The model under review builds one solid part; all positions refer to its coordinate system, in mm. A direction names the side the tool comes from. Give positions to 0.01 mm unless a question says otherwise; leave off trailing zeros. Order: outer loops, then holes, each group sorted by start corner. A loop starts at its lowest first (then second) coordinate and runs counter-clockwise, first axis right, second up. Notation, with made-up numbers: (-4.5, -10) - (36.5, -10) arc R9 ccw to (36.5, -1) - close; hole circle Ø3 at (49, -0.5). An arc over 180 degrees is marked (long way). Use CSV: the item, a comma, the result in double quotes.
```python
from build123d import *

# Parameters (mm, degrees)
SKETCH_1_W          = 300
SKETCH_1_H          = 370
EXTRUDE_1_DEPTH     = 10
SKETCH_2_R          = 1.5
SKETCH_2_R_2        = 2
SKETCH_2_W          = 25
SKETCH_2_H          = 34
CUT_EXTRUDE_1_DEPTH = 10


with BuildPart() as part:
    # 草图1 → 凸台-拉伸1 (new body)
    with BuildSketch(Plane.XY):
        with Locations((113.99815703, 205.554685433)):
            Rectangle(SKETCH_1_W, SKETCH_1_H)
    extrude(amount=EXTRUDE_1_DEPTH)

    # 草图2 → 切除-拉伸1 (cut)
    with BuildSketch(Plane.XY.offset(10)):
        with Locations((253.99815703, 375.554685433)):
            Circle(SKETCH_2_R)
        with Locations((253.99815703, 337.554685433)):
            Circle(SKETCH_2_R)
        with Locations((-26.00184297, 337.554685433)):
            Circle(SKETCH_2_R)
        with Locations((-26.00184297, 375.554685433)):
            Circle(SKETCH_2_R)
        with Locations((-26.00184297, 35.554685433)):
            Circle(SKETCH_2_R)
        with Locations((-26.00184297, 73.554685433)):
            Circle(SKETCH_2_R)
        with Locations((253.99815703, 73.554685433)):
            Circle(SKETCH_2_R)
        with Locations((253.99815703, 35.554685433)):
            Circle(SKETCH_2_R)
        with Locations((237.99815703, 355.804685433)):
            Circle(SKETCH_2_R)
        with Locations((-10.00184297, 355.804685433)):
            Circle(SKETCH_2_R)
        with Locations((-10.00184297, 55.304685433)):
            Circle(SKETCH_2_R)
        with Locations((237.99815703, 55.304685433)):
            Circle(SKETCH_2_R)
        with Locations((237.99815703, 270.554685433)):
            Circle(SKETCH_2_R_2)
        with Locations((257.99815703, 270.554685433)):
            Circle(SKETCH_2_R_2)
        with Locations((257.99815703, 220.554685433)):
            Circle(SKETCH_2_R_2)
        with Locations((-24.980137122, 233.80801348)):
            Circle(SKETCH_2_R_2)
        with Locations((-24.980137122, 283.80801348)):
            Circle(SKETCH_2_R_2)
        with Locations((217.49815703, 373.554685433)):
            Rectangle(SKETCH_2_W, SKETCH_2_H)
        with Locations((10.49815703, 373.554685433)):
            Rectangle(SKETCH_2_W, SKETCH_2_H)
        Polygon((159.455584524, 355.554685433), (159.455584524, 364.554685433), (177.455584524, 364.554685433), (177.455584524, 356.554685433), (177.455584524, 347.554685433), (159.455584524, 347.554685433), align=None)
    extrude(amount=-CUT_EXTRUDE_1_DEPTH, mode=Mode.SUBTRACT)


solid = part.part
```
Item 1: Take a section at B-B, the plane z = 4. State how many separate pieces and enclosed holes the cut face has, and give its area (3 significant figures).
Results list:
separate pieces,"1"
enclosed holes,"18"
area,"109,000 mm2"
Item 2: Take a section at C-C, the plane x = 211. Give the boundary of the cut face in (y, z), and give its area (3 significant figures).
Results list:
outline,"(20.55, 0) - (356.55, 0) - (356.55, 10) - (20.55, 10) - close"
area,"3,360 mm2"
Item 3: Clearance check with a flat-ended pin moving along its axis: pin 1 (2.5 mm diameter, centred on x = -26, y = 337.55, fed in from -Z). State where the tip first meets the part, or that it passes through.
Results list:
pin 1,"passes through"
Item 4: Mouldability with a two-part tool opening along X and no side actions: class faces 4 (the face through (112, 208, 0)), 5 (the face through (229.998, 373, 5)), 6 (the face through (263.998, 203, 5)) as pulls with the +X half, pulls with the -X half, needs draft (parallel to the pull), parting line crosses it, or undercut.
Results list:
face 4,"needs draft"
face 5,"undercut"
face 6,"pulls with the +X half"
Item 5: Wall thickness on L1, parallel to X at y = 356, z = 8.25; L2, parallel to Y at x = 238.5, z = 6.5; L3, parallel to Y at x = 162, z = 5.25: over which ranges is each line inside the solid? List them lowest first.
Results list:
L1,"x = -36 to -11.49, -8.51 to 159.46, 177.46 to 236.51, 239.49 to 264"
L2,"y = 20.55 to 53.89, 56.72 to 268.62, 272.49 to 354.39, 357.22 to 390.55"
L3,"y = 20.55 to 347.55, 364.55 to 390.55"
Item 6: Tool access review of faces 1 (the face through (-2.002, 373, 5)), 2 (the face through (159.456, 356, 5)), 3 (the face through (112, 208, 10)): name each direction out of +Z, -Z, +X, -X, +Y, -Y from which nothing blocks a thin tool from reaching the whole face with its end or side.
Results list:
face 1,"+Z, -Z, +Y"
face 2,"+Z, -Z"
face 3,"+Z, +X, -X, +Y, -Y"
Item 7: Take a section at A-A, the plane x = 170. Give the boundary of the cut face in (y, z), and give its area (3 significant figures).
Results list:
outline,"(20.55, 0) - (347.55, 0) - (347.55, 10) - (20.55, 10) - close; (364.55, 0) - (390.55, 0) - (390.55, 10) - (364.55, 10) - close"
area,"3,530 mm2"
